from build123d import *

# Parameters (mm, degrees)
SKETCH1_W           = 438.1
SKETCH1_H           = 300
BOSS_EXTRUDE1_DEPTH = 12.7
CUT_EXTRUDE1_REACH  = 267.79
SKETCH2_R           = 4
SKETCH2_R_2         = 5
SKETCH3_W           = 3.175
SKETCH3_H           = 205
CUT_EXTRUDE2_DEPTH  = 5
CUT_EXTRUDE3_REACH  = 267.79
SKETCH4_R           = 4
CUT_EXTRUDE4_REACH  = 267.79


with BuildPart() as part:
    # Sketch1 → Boss-Extrude1 (new body)
    with BuildSketch(Plane.XY):
        Rectangle(SKETCH1_W, SKETCH1_H)
    extrude(amount=BOSS_EXTRUDE1_DEPTH)

    # Sketch2 → Cut-Extrude1 (cut, up to next)
    with BuildSketch(Plane.XY.offset(12.7), mode=Mode.PRIVATE) as cut_extrude1_sk1:
        with Locations((76.214870385, 69.409934415)):
            Circle(SKETCH2_R)
    cut_extrude1_tool1 = extrude(cut_extrude1_sk1.sketch, amount=-CUT_EXTRUDE1_REACH, mode=Mode.PRIVATE) & part.part
    # Sketch2 → Cut-Extrude1 (cut, up to next)
    with BuildSketch(Plane.XY.offset(12.7), mode=Mode.PRIVATE) as cut_extrude1_sk2:
        with Locations((76.214870385, 110.590065585)):
            Circle(SKETCH2_R)
    cut_extrude1_tool2 = extrude(cut_extrude1_sk2.sketch, amount=-CUT_EXTRUDE1_REACH, mode=Mode.PRIVATE) & part.part
    # Sketch2 → Cut-Extrude1 (cut, up to next)
    with BuildSketch(Plane.XY.offset(12.7), mode=Mode.PRIVATE) as cut_extrude1_sk3:
        with Locations((99.05, 90)):
            Circle(SKETCH2_R_2)
    cut_extrude1_tool3 = extrude(cut_extrude1_sk3.sketch, amount=-CUT_EXTRUDE1_REACH, mode=Mode.PRIVATE) & part.part
    add(cut_extrude1_tool1.solids().sort_by_distance((76.21487, 69.409934, 12.7))[0], mode=Mode.SUBTRACT)
    add(cut_extrude1_tool2.solids().sort_by_distance((76.21487, 110.590066, 12.7))[0], mode=Mode.SUBTRACT)
    add(cut_extrude1_tool3.solids().sort_by_distance((99.05, 90, 12.7))[0], mode=Mode.SUBTRACT)

    # Sketch3 → Cut-Extrude2 (cut)
    with BuildSketch(Plane.XY.offset(12.7)):
        with Locations((-209.525, 47.5)):
            Rectangle(SKETCH3_W, SKETCH3_H)
    extrude(amount=-CUT_EXTRUDE2_DEPTH, mode=Mode.SUBTRACT)

    # Sketch4 → Cut-Extrude3 (cut, up to next)
    with BuildSketch(Plane.XY.offset(12.7), mode=Mode.PRIVATE) as cut_extrude3_sk1:
        with Locations((-180.95, -75)):
            Circle(SKETCH4_R)
    cut_extrude3_tool1 = extrude(cut_extrude3_sk1.sketch, amount=-CUT_EXTRUDE3_REACH, mode=Mode.PRIVATE) & part.part
    # Sketch4 → Cut-Extrude3 (cut, up to next)
    with BuildSketch(Plane.XY.offset(12.7), mode=Mode.PRIVATE) as cut_extrude3_sk2:
        with Locations((-180.95, -125)):
            Circle(SKETCH4_R)
    cut_extrude3_tool2 = extrude(cut_extrude3_sk2.sketch, amount=-CUT_EXTRUDE3_REACH, mode=Mode.PRIVATE) & part.part
    # Sketch4 → Cut-Extrude3 (cut, up to next)
    with BuildSketch(Plane.XY.offset(12.7), mode=Mode.PRIVATE) as cut_extrude3_sk3:
        with Locations((180.95, -125)):
            Circle(SKETCH4_R)
    cut_extrude3_tool3 = extrude(cut_extrude3_sk3.sketch, amount=-CUT_EXTRUDE3_REACH, mode=Mode.PRIVATE) & part.part
    # Sketch4 → Cut-Extrude3 (cut, up to next)
    with BuildSketch(Plane.XY.offset(12.7), mode=Mode.PRIVATE) as cut_extrude3_sk4:
        with Locations((180.95, -75)):
            Circle(SKETCH4_R)
    cut_extrude3_tool4 = extrude(cut_extrude3_sk4.sketch, amount=-CUT_EXTRUDE3_REACH, mode=Mode.PRIVATE) & part.part
    add(cut_extrude3_tool1.solids().sort_by_distance((-180.95, -75, 12.7))[0], mode=Mode.SUBTRACT)
    add(cut_extrude3_tool2.solids().sort_by_distance((-180.95, -125, 12.7))[0], mode=Mode.SUBTRACT)
    add(cut_extrude3_tool3.solids().sort_by_distance((180.95, -125, 12.7))[0], mode=Mode.SUBTRACT)
    add(cut_extrude3_tool4.solids().sort_by_distance((180.95, -75, 12.7))[0], mode=Mode.SUBTRACT)

    # Sketch5 → Cut-Extrude4 (cut, up to next)
    with BuildSketch(Plane.XY.offset(12.7), mode=Mode.PRIVATE) as cut_extrude4_sk1:
        with BuildLine():
            Line((15, 95), (-75, 95))
            ThreePointArc((-75, 95), (-90, 110), (-75, 125))
            Line((-75, 125), (15, 125))
            ThreePointArc((15, 125), (30, 110), (15, 95))
        make_face()
    cut_extrude4_tool1 = extrude(cut_extrude4_sk1.sketch, amount=-CUT_EXTRUDE4_REACH, mode=Mode.PRIVATE) & part.part
    add(cut_extrude4_tool1.solids().sort_by_distance((-30, 110, 12.7))[0], mode=Mode.SUBTRACT)


solid = part.part
Verification items for the finished model (mm, model axes). A direction names the side the tool comes from. Give positions to 0.01 mm unless a question says otherwise; leave off trailing zeros. Loops run counter-clockwise (first coordinate to the right, second up) from the corner with the lowest first, then second, coordinate; pieces in that order, holes last. Notation, with made-up numbers: (26.5, 48.5) - (67.5, 48.5) arc R23 cw to (67.5, 84.5) - close; hole circle Ø10 at (13.5, 60). An arc over 180 degrees is marked (long way). Write each question's results on one line, items separated by ' | '.
1) Sectioned sample at A-A on x = -23. Record the boundary of the cut face in (y, z), plus the area to 3 significant figures.
Solution:
outline: (-150, 0) - (95, 0) - (95, 12.7) - (-150, 12.7) - close; (125, 0) - (150, 0) - (150, 12.7) - (125, 12.7) - close | area: 3,430 mm2
2) Sectioned sample at C-C on z = 9.75. Count the separate pieces of the cut face and the enclosed holes in it, plus the area to 3 significant figures.
Solution:
separate pieces: 1 | enclosed holes: 8 | area: 127,000 mm2
3) Material ranges on L1, parallel to Y at x = 180.95, z = 7.25; L2, parallel to X at y = -34, z = 12; L3, parallel to Y at x = 99.05, z = 5.25, recorded low to high. Write a range as from..to.
Solution:
L1: -150..-129, -121..-79, -71..150 | L2: -219.05..-211.11, -207.94..219.05 | L3: -150..85, 95..150
4) Mould release check, pull along X, two halves, no side actions. Record for faces 1 (the flat face through (-219.05, -2, 6)), 2 (the cylindrical face through (177.776, -77.434, 6.439)), 3 (the flat face through (-3, 150, 6)): pulls with the +X half, pulls with the -X half, needs draft (parallel to the pull), parting line crosses it, or undercut.
Solution:
face 1: pulls with the -X half | face 2: undercut | face 3: needs draft
5) Depth check by flat-ended pin: P1, Ø9, axis at x = -180.95, y = -75, coming from the +Z side; P2, Ø1.6, axis at x = -210, y = 0.5, coming from the +Z side. Enter the tip coordinate at first touch or a pass-through.
Solution:
P1: z = 12.7 | P2: z = 7.7
6) Tool access check on faces 4 (the cylindrical face through (-90, 110, 6)), 5 (the flat face through (-3, 2, 12.7)). Record the directions out of +Z, -Z, +X, -X, +Y, -Y that give a thin tool (end or side, any length) a straight path to the whole face; none if there is none.
Solution:
face 4: +Z, -Z | face 5: +Z, +X, -X, +Y, -Y
7) Sectioned sample at B-B on y = 90. Record the boundary of the cut face in (x, z), plus the area to 3 significant figures.
Solution:
outline: (-219.05, 0) - (94.05, 0) - (94.05, 12.7) - (-207.94, 12.7) - (-207.94, 7.7) - (-211.11, 7.7) - (-211.11, 12.7) - (-219.05, 12.7) - close; (104.05, 0) - (219.05, 0) - (219.05, 12.7) - (104.05, 12.7) - close | area: 5,420 mm2
